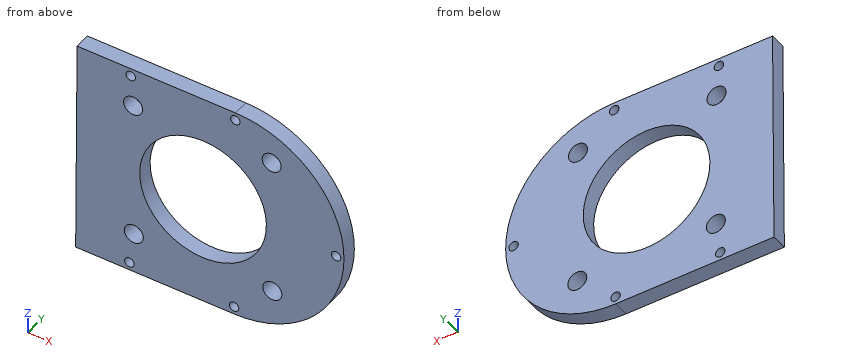
from build123d import *

# Parameters (mm, degrees)
SKETCH1_R           = 20
SKETCH1_R_2         = 3
SKETCH1_R_3         = 1.5
BOSS_EXTRUDE1_DEPTH = 5


with BuildPart() as part:
    # Sketch1 → Boss-Extrude1 (new body)
    with BuildSketch(Plane(origin=(0, 0, 0), x_dir=(1, 0, 0), z_dir=(0, 1, 0))):
        with BuildLine():
            Line((204.265004565, -121.165074652), (154.266061792, -121.490223172))
            Line((154.266061792, -121.490223172), (154.714766749, -190.488764199))
            Line((154.714766749, -190.488764199), (204.713709523, -190.163615679))
            ThreePointArc((204.713709523, -190.163615679), (238.988627557, -155.439992687), (204.265004565, -121.165074652))
        make_face()
        with Locations(Location((194.489996124, -155.990223157, 0), (0, 0, 270))):
            Circle(SKETCH1_R, mode=Mode.SUBTRACT)
        with Locations(Location((216.371480989, -134.502016601, 0), (0, 0, 270))):
            Circle(SKETCH1_R_2, mode=Mode.SUBTRACT)
        with Locations(Location((171.23195345, -123.879945011, 0), (0, 0, 270))):
            Circle(SKETCH1_R_3, mode=Mode.SUBTRACT)
        with Locations(Location((204.281261991, -123.665021791, 0), (0, 0, 270))):
            Circle(SKETCH1_R_3, mode=Mode.SUBTRACT)
        with Locations(Location((236.488680419, -155.456250113, 0), (0, 0, 270))):
            Circle(SKETCH1_R_3, mode=Mode.SUBTRACT)
        with Locations(Location((171.648143556, -187.87859176, 0), (0, 0, 270))):
            Circle(SKETCH1_R_3, mode=Mode.SUBTRACT)
        with Locations(Location((204.697452097, -187.663668541, 0), (0, 0, 270))):
            Circle(SKETCH1_R_3, mode=Mode.SUBTRACT)
        with Locations(Location((216.155888878, -178.252189218, 0), (0, 0, 270))):
            Circle(SKETCH1_R_2, mode=Mode.SUBTRACT)
        with Locations(Location((172.405716262, -178.036597107, 0), (0, 0, 270))):
            Circle(SKETCH1_R_2, mode=Mode.SUBTRACT)
        with Locations(Location((172.621308373, -134.286424491, 0), (0, 0, 270))):
            Circle(SKETCH1_R_2, mode=Mode.SUBTRACT)
    extrude(amount=BOSS_EXTRUDE1_DEPTH)


solid = part.part
Can you work these out from the model? Positions are in its coordinate system, mm. Round coordinates to 2 decimals unless told otherwise and drop trailing zeros. Write each loop counter-clockwise with the first axis right and the second up, starting at its lowest first coordinate (ties: lowest second). Pieces come first, ordered by that corner, then holes. Notation, with made-up numbers: M -4,57 L 9,57 A30 cw 9,93 Z; hole C 40,-14 d10. An arc over 180 degrees is marked long. Use CSV: the item, a comma, the result in double quotes.
(1) Imagine slicing it at C-C (y = 1.4). Count the separate pieces of the cut face and the enclosed holes in it, plus the area to 3 significant figures.
Check values:
separate pieces,"1"
enclosed holes,"10"
area,"3,910 mm^2"
(2) Imagine slicing it at A-A (x = 198). Write out the boundary of the cut face in (y, z), plus the area to 3 significant figures.
Check values:
outline,"M 0,121.21 L 5,121.21 L 5,136.3 L 0,136.3 Z; M 0,175.68 L 5,175.68 L 5,190.21 L 0,190.21 Z"
area,"148 mm^2"
(3) Imagine slicing it at D-D (z = 155). Write out the boundary of the cut face in (x, y), plus the area to 3 significant figures.
Check values:
outline,"M 154.48,0 L 174.51,0 L 174.51,5 L 154.48,5 Z; M 214.47,0 L 235.06,0 L 235.06,5 L 214.47,5 Z; M 237.92,0 L 238.98,0 L 238.98,5 L 237.92,5 Z"
area,"208 mm^2"
(4) I'm going to push flat-ended pins straight in: pin 1 (1 mm diameter, centred on x = 192.5, y = 1.5, fed in from +Z); pin 2 (2.5 mm diameter, centred on x = 171.65, z = 187.88, fed in from -Y); pin 3 (3 mm diameter, centred on y = 3, z = 132, fed in from +X); pin 4 (1 mm diameter, centred on y = 1, z = 131, fed in from +X). Where does each tip first touch, or does it pass through?
Check values:
pin 1,"z = 190.25"
pin 2,"through"
pin 3,"x = 230.93"
pin 4,"x = 229.11"
(5) I need wall thicknesses on line 1 along X through (y, z) = (2.95, 178); line 2 along Z through (x, y) = (203.5, 4.1); line 3 along Z through (x, y) = (171, 2.05). Which ranges of each line are inside material? Lowest first, please.
Check values:
line 1,"154.63 to 169.41, 175.41 to 213.17, 219.15 to 230.78"
line 2,"121.17 to 122.38, 124.95 to 138.13, 173.85 to 186.76, 188.57 to 190.17"
line 3,"121.38 to 122.4, 125.36 to 131.76, 136.81 to 175.39, 180.69 to 186.53, 189.23 to 190.38"
(6) Imagine slicing it at B-B (z = 141.5). Write out the boundary of the cut face in (x, y).
Check values:
outline,"M 154.4,0 L 180.7,0 L 180.7,5 L 154.4,5 Z; M 208.28,0 L 235.95,0 L 235.95,5 L 208.28,5 Z"
